Can you work these out from the model? Positions are in its coordinate system, mm. Face numbers are marked on the shaded views. A direction names the side the tool comes from. Give positions to 0.01 mm unless a question says otherwise; leave off trailing zeros. Loops run counter-clockwise (first coordinate to the right, second up) from the corner with the lowest first, then second, coordinate; pieces in that order, holes last. Notation, with made-up numbers: (21.5, 81.25) - (62.5, 81.25) arc R20 cw to (62.5, 107.25) - close; hole circle Ø2 at (34, -26.5). An arc over 180 degrees is marked (long way). Write item = value, one per line.
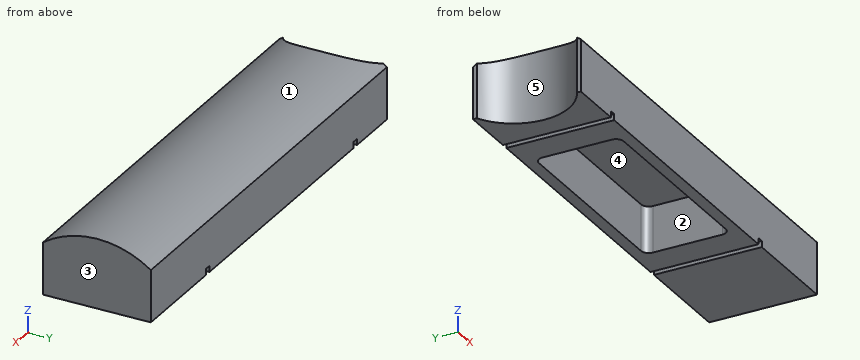
from build123d import *

# Parameters (mm, degrees)
F0_W          = 177.8
F0_H          = 31.75
F11_DEPTH     = 22.225
F1_W          = 2.54
F1_H          = 2.54
F2_DEPTH      = 22.225
F2_DEPTH_BACK = 22.225
F4_DEPTH      = 31.751
F6_DEPTH      = 177.801
F7_W          = 83.185
F7_H          = 34.925
F8_DEPTH      = 19.05
F9_R          = 3.175


with BuildPart() as f11:
    # F0 (on Front) → F11 (new body, symmetric)
    with BuildSketch(Plane.XZ):
        Rectangle(F0_W, F0_H)
    extrude(amount=F11_DEPTH, both=True)

    # F1 (on Front) → F2 (cut, two sides)
    with BuildSketch(Plane.XZ) as f2_sk:
        with Locations((-65.0875, -14.605)):
            Rectangle(F1_W, F1_H)
        with Locations((46.0375, -14.605)):
            Rectangle(F1_W, F1_H)
    extrude(amount=F2_DEPTH, mode=Mode.SUBTRACT)
    extrude(f2_sk.sketch, amount=-F2_DEPTH_BACK, mode=Mode.SUBTRACT)

    # F3 (on face) → F4 (cut, through all)
    with BuildSketch(Plane.XY.offset(15.875)):
        with BuildLine():
            Line((-88.9, 20.6375), (-88.9, -20.6375))
            ThreePointArc((-88.9, -20.6375), (-76.2, 0), (-88.9, 20.6375))
        make_face()
    extrude(amount=-F4_DEPTH, mode=Mode.SUBTRACT)

    # F5 (on face) → F6 (cut, through all)
    with BuildSketch(Plane.YZ.offset(88.9)):
        with BuildLine():
            ThreePointArc((-22.225, 5.546072), (0, 12.7), (22.225, 5.546072))
            Line((22.225, 5.546072), (22.225, 15.875))
            Line((22.225, 15.875), (-22.225, 15.875))
            Line((-22.225, 15.875), (-22.225, 5.546072))
        make_face()
    extrude(amount=-F6_DEPTH, mode=Mode.SUBTRACT)

    # F7 (on face) → F8 (cut)
    with BuildSketch(Plane(origin=(0, 0, -15.875), x_dir=(1, 0, 0), z_dir=(0, 0, -1))):
        with Locations((-9.525, 0)):
            Rectangle(F7_W, F7_H)
    extrude(amount=-F8_DEPTH, mode=Mode.SUBTRACT)

    # F9
    f9_edges = [f11.edges().sort_by_distance(p)[0] for p in [
        (32.0675, -17.4625, -6.35),
        (-51.1175, -17.4625, -6.35),
        (-51.1175, 17.4625, -6.35),
        (32.0675, 17.4625, -6.35),
    ]]
    fillet(f9_edges, radius=F9_R)


solid = f11.part
Q1. I need wall thicknesses on L1, parallel to Y at x = -44, z = -10 (1 decimal); L2, parallel to X at y = -15, z = -14; L3, parallel to Z at x = 3, y = 0 (3 decimals). Which ranges of each line are inside material? Lowest first, please.
Output:
L1 = -22.2 to -17.5, 17.5 to 22.2
L2 = -81.73 to -66.36, -63.82 to -51.04, 31.99 to 44.77, 47.31 to 88.9
L3 = 3.175 to 12.7
Q2. Imagine slicing it at C-C, the plane y = 8. Write out the boundary of the cut face in (x, z) (1 decimal), then the cut area to 3 significant figures.
Output:
outline = (-77.6, -15.9) - (-66.4, -15.9) - (-66.4, -13.3) - (-63.8, -13.3) - (-63.8, -15.9) - (-51.1, -15.9) - (-51.1, 3.2) - (32.1, 3.2) - (32.1, -15.9) - (44.8, -15.9) - (44.8, -13.3) - (47.3, -13.3) - (47.3, -15.9) - (88.9, -15.9) - (88.9, 11.9) - (-77.6, 11.9) - close
area = 3,020 mm2
Q3. Imagine slicing it at B-B, the plane x = -3.5. Write out the boundary of the cut face in (y, z) (1 decimal), then the cut area to 3 significant figures.
Output:
outline = (-22.2, -15.9) - (-17.5, -15.9) - (-17.5, 3.2) - (17.5, 3.2) - (17.5, -15.9) - (22.2, -15.9) - (22.2, 5.5) arc R38.1 ccw to (-22.2, 5.5) - close
area = 503 mm2
Q4. Which directions (+Z, -Z, +X, -X, +Y, -Y) give clear straight access to the entire face, cutting with the end or side of a thin tool? Please do the marked faces 4 and 5.
Output:
face_4 = -Z
face_5 = +Z, -Z, -X
Q5. For pin 1 (4 mm diameter, centred on y = 12, z = 4.5, fed in from -X); pin 2 (4 mm diameter, centred on x = -4, y = -8.5, fed in from +Z); pin 3 (2 mm diameter, centred on y = 0.5, z = -15, fed in from -X), each with a flat end and sliding along its axis, tell me the tip position at first contact or that it passes through.
Output:
pin_1 = -80.92
pin_2 = 12.14
pin_3 = -76.25
Q6. We'd pull the mould along X, two halves only. Please class the marked faces 1, 2 and 3: released by +X, released by -X, zero draft, split by the parting line, or undercut.
Output:
face_1 = zero draft
face_2 = undercut
face_3 = released by +X
Q7. Imagine slicing it at D-D, the plane z = 10.5. Write out the boundary of the cut face in (x, y).
Output:
outline = (-80.04, -12.76) - (88.9, -12.76) - (88.9, 12.76) - (-80.04, 12.76) arc R23.12 cw to start
